Build history of the part. All positions in model axes, mm. A direction names the side the tool comes from. Coordinates: 2 decimals unless noted, no trailing zeros. Loops run counter-clockwise (first coordinate to the right, second up) from the corner with the lowest first, then second, coordinate; pieces in that order, holes last.
(1) Slice it at D-D (z = -55). Give the cut face in (x, y) (3 decimals), and give its area (3 significant figures).
(2) Slice it at A-A (y = 6). Give the cut face in (x, z), and give its area (3 significant figures).
(3) Slice it at B-B (x = 88.2). Give the cut face in (y, z) (3 decimals), and give its area (3 significant figures).
(4) Flat gauge pins, fed straight in: P1, Ø7.5, axis at x = 94, z = -43, coming from the -Y side (3 decimals); P2, Ø1.2, axis at x = -3, y = 9, coming from the +Z side; P3, Ø6, axis at x = 83.5, y = 7, coming from the -Z side; P4, Ø8, axis at x = 66.5, y = 2, coming from the +Z side. Where does each tip first touch, or does it go through?
(5) Slice it at C-C (z = -38.1). Give the cut face in (x, y) (3 decimals).
(6) Wall check: L1, parallel to X at y = 8.8, z = -38.1; L2, parallel to X at y = 8.5, z = -24; L3, parallel to X at y = 11.75, z = -59. Give the ranges that are in metal, low to high.
(7) Tool access for faces 1 (the face through (89, 5, -12.7)), 2 (the face through (89, 5, -63.5)), 3 (the face through (73.66, 9, -38)): list every direction of +Z, -Z, +X, -X, +Y, -Y with a clear straight run to the whole face (end or side of a thin tool).
(8) Two-plate mould, pull along Z, no slides. Class faces 4 (the face through (-2, 8, -12.7)), 5 (the face through (2.54, 9, -38)), 6 (the face through (101.6, 9, -38)): pulls with the +Z half, pulls with the -Z half, needs draft (parallel to the pull), parting line crosses it, or undercut.
from build123d import *

# Parameters (mm, degrees)
SKETCH1_W           = 76.2
SKETCH1_H           = 76.2
BOSS_EXTRUDE1_DEPTH = 2.54
SKETCH2_W           = 76.2
SKETCH2_H           = 76.2
SKETCH2_W_2         = 71.12
SKETCH2_H_2         = 71.12
BOSS_EXTRUDE2_DEPTH = 12.7
SKETCH3_W           = 50.8
SKETCH3_H           = 2.54
BOSS_EXTRUDE3_DEPTH = 25.4
SKETCH5_R           = 3
CUT_EXTRUDE2_DEPTH  = 11.795
SKETCH6_W           = 25.4
SKETCH6_H           = 2.54
BOSS_EXTRUDE4_DEPTH = 8.255
SKETCH9_W           = 50.8
SKETCH9_H           = 2.54
BOSS_EXTRUDE5_DEPTH = 1.5
SKETCH10_W          = 50.8
SKETCH10_H          = 15.24
BOSS_EXTRUDE6_DEPTH = 2.54


with BuildPart() as part:
    # Sketch1 → Boss-Extrude1 (new body)
    with BuildSketch(Plane(origin=(0, 0, 0), x_dir=(1, 0, 0), z_dir=(0, 1, 0))):
        with Locations((38.1, 38.1)):
            Rectangle(SKETCH1_W, SKETCH1_H)
    extrude(amount=BOSS_EXTRUDE1_DEPTH)

    # Sketch2 → Boss-Extrude2 (add)
    with BuildSketch(Plane(origin=(0, 2.54, 0), x_dir=(1, 0, 0), z_dir=(0, 1, 0))):
        with Locations((38.1, 38.1)):
            Rectangle(SKETCH2_W, SKETCH2_H)
        with Locations((38.1, 38.1)):
            Rectangle(SKETCH2_W_2, SKETCH2_H_2, mode=Mode.SUBTRACT)
    extrude(amount=BOSS_EXTRUDE2_DEPTH)

    # Sketch3 → Boss-Extrude3 (add)
    with BuildSketch(Plane(origin=(76.2, 0, 0), x_dir=(0, 0, -1), z_dir=(1, 0, 0))):
        with Locations((38.1, 9.525)):
            Rectangle(SKETCH3_W, SKETCH3_H)
    extrude(amount=BOSS_EXTRUDE3_DEPTH)

    # Sketch5 → Cut-Extrude2 (cut, through all)
    with BuildSketch(Plane(origin=(0, 10.795, 0), x_dir=(1, 0, 0), z_dir=(0, 1, 0))):
        with Locations((88.2, 38.1)):
            Circle(SKETCH5_R)
    extrude(amount=-CUT_EXTRUDE2_DEPTH, mode=Mode.SUBTRACT)

    # Sketch6 → Boss-Extrude4 (add)
    with BuildSketch(Plane.XZ.offset(-8.255)):
        with Locations((88.9, -13.97)):
            Rectangle(SKETCH6_W, SKETCH6_H)
        with Locations((88.9, -62.23)):
            Rectangle(SKETCH6_W, SKETCH6_H)
    extrude(amount=BOSS_EXTRUDE4_DEPTH)

    # Sketch9 → Boss-Extrude5 (add)
    with BuildSketch(Plane.ZY):
        with Locations((-38.1, 1.27)):
            Rectangle(SKETCH9_W, SKETCH9_H)
    extrude(amount=BOSS_EXTRUDE5_DEPTH)

    # Sketch10 → Boss-Extrude6 (add)
    with BuildSketch(Plane.ZY.offset(1.5)):
        with Locations((-38.1, 7.62)):
            Rectangle(SKETCH10_W, SKETCH10_H)
    extrude(amount=BOSS_EXTRUDE6_DEPTH)


solid = part.part
Response values:
1. outline: (-4.04, 0) - (76.2, 0) - (76.2, 8.255) - (101.6, 8.255) - (101.6, 10.795) - (76.2, 10.795) - (76.2, 15.24) - (73.66, 15.24) - (73.66, 2.54) - (2.54, 2.54) - (2.54, 15.24) - (0, 15.24) - (0, 2.54) - (-1.5, 2.54) - (-1.5, 15.24) - (-4.04, 15.24) - close
1. area: 365 mm2
2. outline: (-4.04, -63.5) - (-1.5, -63.5) - (-1.5, -12.7) - (-4.04, -12.7) - close; (0, -76.2) - (76.2, -76.2) - (76.2, -63.5) - (101.6, -63.5) - (101.6, -60.96) - (76.2, -60.96) - (76.2, -15.24) - (101.6, -15.24) - (101.6, -12.7) - (76.2, -12.7) - (76.2, 0) - (0, 0) - close; hole (2.54, -73.66) - (73.66, -73.66) - (73.66, -2.54) - (2.54, -2.54) - close
2. area: 1,010 mm2
3. outline: (0, -63.5) - (10.795, -63.5) - (10.795, -41.1) - (8.255, -41.1) - (8.255, -60.96) - (0, -60.96) - close; (0, -15.24) - (8.255, -15.24) - (8.255, -35.1) - (10.795, -35.1) - (10.795, -12.7) - (0, -12.7) - close
3. area: 156 mm2
4. P1: stops at y = 8.255
4. P2: stops at z = -12.7
4. P3: stops at z = -63.5
4. P4: stops at z = 0
5. outline: (-4.04, 0) - (76.2, 0) - (76.2, 8.255) - (85.2, 8.255) - (85.2, 10.795) - (76.2, 10.795) - (76.2, 15.24) - (73.66, 15.24) - (73.66, 2.54) - (2.54, 2.54) - (2.54, 15.24) - (0, 15.24) - (0, 2.54) - (-1.5, 2.54) - (-1.5, 15.24) - (-4.04, 15.24) - close; (91.2, 8.255) - (101.6, 8.255) - (101.6, 10.795) - (91.2, 10.795) - close
6. L1: x = -4.04 to -1.5, 0 to 2.54, 73.66 to 85.2, 91.2 to 101.6
6. L2: x = -4.04 to -1.5, 0 to 2.54, 73.66 to 101.6
6. L3: x = -4.04 to -1.5, 0 to 2.54, 73.66 to 76.2
7. face 1: +Z, +X, +Y, -Y
7. face 2: -Z, +X, +Y, -Y
7. face 3: +Y
8. face 4: pulls with the +Z half
8. face 5: undercut
8. face 6: needs draft
